```python
from build123d import *

# Parameters (mm, degrees)
F2_R = 9.525
F4_R = 5.08


# Not quite as in the source:
# - a fillet or chamfer that OpenCascade refuses, or shapes differently, is made with other operations: its cross-section is extruded or revolved along the edge and cut away or added


with BuildPart() as f1:
    # F0 (on Front) → F1 (revolve)
    with BuildSketch(Plane.XZ):
        Polygon((0, 4.7625), (0, 0), (64.516, 0), (64.516, 9.525), (8.89, 9.525), (8.89, 4.7625), align=None)
    revolve(axis=Axis((32.258, 0, 0), (-1, 0, 0)))

    # F2
    f2_edges = [f1.edges().sort_by_distance(p)[0] for p in [
        (64.516, 0, -9.525),
    ]]
    fillet(f2_edges, radius=F2_R)

    # F3: fillet of radius 5.08 on 1 edges, made by hand

    # F3_s1 → F3_t2 (revolve, cut)
    with BuildSketch(Plane.XZ):
        with BuildLine():
            ThreePointArc((13.9600684167, 9.525), (10.4820301765, 8.1476544532), (8.89, 4.7625))
            Line((8.89, 4.7625), (8.89, 9.525))
            Line((8.89, 9.525), (13.9600684167, 9.525))
        make_face()
    revolve(axis=Axis((8.89, 0, 0), (-1, 0, 0)), mode=Mode.SUBTRACT)

    # F4
    f4_edges = [f1.edges().sort_by_distance(p)[0] for p in [
        (8.89, 0, -4.7625),
    ]]
    fillet(f4_edges, radius=F4_R)


solid = f1.part
```
Build history of the part. All positions in model axes, mm. A direction names the side the tool comes from. Give positions to 0.01 mm unless a question says otherwise; leave off trailing zeros. Loops run counter-clockwise (first coordinate to the right, second up) from the corner with the lowest first, then second, coordinate; pieces in that order, holes last. Notation, with made-up numbers: (-39.75, 85.5) -> (17.25, 85.5) arc R22 ccw to (17.25, 97.5) -> close; hole circle Ø1 at (88, 63). An arc over 180 degrees is marked (long way). One line per question, with ' | ' between items. Start each with the question number.
1) Pin check, flat tips, straight feed: pin 1 (1.5 mm diameter, centred on x = 49, y = -6.5, fed in from +Z); pin 2 (1.5 mm diameter, centred on x = 38.5, z = -2.5, fed in from -Y); pin 3 (1.5 mm diameter, centred on x = 33.5, y = 3.5, fed in from +Z). Stop position of each tip, or through.
2) Cut at A-A (x = 26.5). Give the cut face in (y, z) (3 decimals), plus the area to 3 significant figures.
3) Probe L1, parallel to Z at x = 28, y = -6; L2, parallel to Y at x = 9, z = -5.25; L3, parallel to Z at x = 6, y = -1.5. List the from-to ranges inside material, lowest first.
4) 3-axis set-ups, long thin cutter, end or side, ignore diameter. For faces 1 (the cylindrical face through (2.64, -1.82, 4.4)), 2 (the flat face through (0, 0, 0)): which of +Z, -Z, +X, -X, +Y, -Y reach the whole face in a straight line?
5) Cut at B-B (x = 57.5). Give the cut face in (y, z).
Return value:
1) pin 1: z = 7.59 | pin 2: y = -9.36 | pin 3: z = 9.12
2) outline: circle Ø19.05 at (0, 0) | area: 285 mm^2
3) L1: -7.4 to 7.4 | L2: -3.49 to 3.49 | L3: -4.56 to 4.56
4) face 1: -X | face 2: +Z, -Z, -X, +Y, -Y
5) outline: circle Ø18.38 at (0, 0)
